```python
from build123d import *

# Parameters (mm, degrees)
BOX088_W                  = 7.5
BOX088_H                  = 1
BOX088_DEPTH              = 1
BOX087_W                  = 7.5
BOX087_H                  = 1
BOX087_DEPTH              = 1
FUSION017_PLACEMENT_ANGLE = 45


with BuildPart() as cube088:
    # Box088 → Box088 (new body)
    with BuildSketch(Plane.XY):
        with Locations((3.75, 0.5)):
            Rectangle(BOX088_W, BOX088_H)
    extrude(amount=BOX088_DEPTH)


with BuildPart() as obj1:
    # Box087 → Box087 (new body)
    with BuildSketch(Plane(origin=(1, 0, 0), x_dir=(0, 1, 0), z_dir=(0, 0, 1))):
        with Locations((3.75, 0.5)):
            Rectangle(BOX087_W, BOX087_H)
    extrude(amount=BOX087_DEPTH)

    # Fusion017: union Cube088
    add(cube088.part)


with BuildPart() as obj1_1:
    # Fusion017 placement: moved
    add(obj1.part.moved(Location((0, -15, 0))).rotate(Axis((0, -15, 0), (0, 0, 1)), FUSION017_PLACEMENT_ANGLE))


solid = obj1_1.part
```
The model under review builds one solid part; all positions refer to its coordinate system, in mm. Give positions to 0.01 mm unless a question says otherwise; leave off trailing zeros. Write each loop counter-clockwise with the first axis right and the second up, starting at its lowest first coordinate (ties: lowest second). Pieces come first, ordered by that corner, then holes. Notation, with made-up numbers: (33.5, 84) - (37.5, 84) arc R21 cw to (37.5, 117) - close; hole circle Ø5 at (24.25, 55.5). An arc over 180 degrees is marked (long way). Answer in a Markdown table with one row per item. Add a question column.
1. Draft analysis for pull direction X (two halves, no side actions). For faces 1 (the flat face through (-2.6, -12.4, 0.5)), 2 (the flat face through (2.266, -11.32, 0.493)), 3 (the flat face through (-2.266, -11.32, 0.493)), 4 (the flat face through (2.7, -12.3, 0.5)), state which applies: +X half, -X half, draft (parallel to the pull), parting line (faces both ways), or undercut.
2. We need section C-C on x = 1. Write out the cut boundary in (y, z), then the cut area to 3 significant figures.
3. Wall thickness on line 1 along X through (y, z) = (-10.5, 0.25); line 2 along X through (y, z) = (-10, 0.75); line 3 along Y through (x, z) = (-2.75, 0.75): over which ranges is each line inside the solid? List them lowest first. Write a range as [from, to].
4. We need section A-A on y = -12.75. Write out the cut boundary in (x, z).
5. We need section B-B on z = 0.35. Write out the cut boundary in (x, y).
Ans:
| question | item | result |
|---|---|---|
| 1 | face 1 | -X half |
| 1 | face 2 | undercut |
| 1 | face 3 | undercut |
| 1 | face 4 | +X half |
| 2 | outline | (-14, 0) - (-12.59, 0) - (-12.59, 1) - (-14, 1) - close |
| 2 | area | 1.41 mm^2 |
| 3 | line 1 | x = [-4.5, -3.09], [3.09, 4.5] |
| 3 | line 2 | x = [-5, -3.59], [3.59, 5] |
| 3 | line 3 | y = [-12.25, -10.84] |
| 4 | outline | (-2.25, 0) - (-0.84, 0) - (-0.84, 1) - (-2.25, 1) - close; (0.84, 0) - (2.25, 0) - (2.25, 1) - (0.84, 1) - close |
| 5 | outline | (-5.3, -9.7) - (0, -15) - (5.3, -9.7) - (4.6, -8.99) - (0, -13.59) - (-4.6, -8.99) - close |
